```python
from build123d import *


with BuildPart() as f1:
    # F0 (on Front) → F1 (revolve)
    with BuildSketch(Plane.XZ):
        Polygon((0, 12.978721), (0, 0), (23.66708, 0), (23.66708, 56.037541), (65.809757, 64.282842), (65.809757, 75.581968), (50.235286, 75.581968), (-27.942425, 64.282842), (-27.942425, 56.037541), (0, 56.037541), (0, 47.486853), (-27.942425, 47.486853), (-27.942425, 39.546926), (0, 39.546926), (0, 30.080097), (-6.565706, 30.080097), (-6.565706, 21.224026), (-31.301621, 21.224026), (-31.301621, 12.978721), align=None)
    revolve(axis=Axis((11.83354, 0, 0), (-1, 0, 0)))


solid = f1.part
```
Read the model definition and answer for the solid it produces. Units are mm, in the model's axes. A direction names the side the tool comes from. Round coordinates to 2 decimals unless told otherwise and drop trailing zeros. Loops run counter-clockwise (first coordinate to the right, second up) from the corner with the lowest first, then second, coordinate; pieces in that order, holes last. Notation, with made-up numbers: (85.5, -37) -> (140.5, -37) arc R17 cw to (140.5, -29) -> close; hole circle Ø11 at (38.25, -28.5). An arc over 180 degrees is marked (long way). One line per item, written item: value.
1) Consider L1, parallel to Y at x = -11.75, z = 0; L2, parallel to Y at x = -7, z = -4.5; L3, parallel to Z at x = -26.5, y = 23. Determine where each line is inside the solid, lowest interval first. Write a range as [from, to].
Answer list:
L1: y = [-66.62, -56.04], [-47.49, -39.55], [-21.22, -12.98], [12.98, 21.22], [39.55, 47.49], [56.04, 66.62]
L2: y = [-67.16, -55.86], [-47.27, -39.29], [-20.74, -12.17], [12.17, 20.74], [39.29, 47.27], [55.86, 67.16]
L3: z = [-60.25, -51.1], [-41.55, -32.17], [32.17, 41.55], [51.1, 60.25]
2) The mould has two halves that part along Y. Classify faces 4 (the face through (-13.8, -38.6, -8.6)), 5 (the face through (-31.302, -9, -10)), 6 (the face through (57.914, -73.785, -16.385)): pulls with the +Y half, pulls with the -Y half, needs draft (parallel to the pull), parting line crosses it, or undercut.
Answer list:
face 4: undercut
face 5: needs draft
face 6: parting line crosses it
3) A cutting plane is placed at D-D (x = 14). Determine the outline of the cut face in (y, z), and give its area (3 significant figures).
Answer list:
outline: circle Ø140.69 at (0, 0)
area: 15,500 mm²
4) A cutting plane is placed at A-A (x = -12). Determine the outline of the cut face in (y, z), and give its area (3 significant figures).
Answer list:
outline: circle Ø133.17 at (0, 0); circle Ø94.97 at (0, 0); circle Ø42.45 at (0, 0); hole circle Ø112.08 at (0, 0); hole circle Ø79.09 at (0, 0); hole circle Ø25.96 at (0, 0)
area: 7,120 mm²
5) Flat-ended cylindrical pins translate along their axes: P1, Ø5, axis at x = 45.5, y = 17.5, coming from the -Z side; P2, Ø10, axis at x = -17.5, y = -25.5, coming from the +Z side; P3, Ø12, axis at y = -28, z = 30, coming from the -X side. Find the tip coordinate at first contact, or state that the pin passes through.
Answer list:
P1: stops at z = -73.5
P2: stops at z = 62.68
P3: stops at x = -27.94
6) For faces 1 (the face through (0, 13, -46)), 2 (the face through (65.81, 51, 40)), 3 (the face through (23.667, 1, 1)), determine the directions among +Z, -Z, +X, -X, +Y, -Y from which every point of the face is accessible in a straight line to the end or side of a thin tool.
Answer list:
face 1: -X
face 2: +Z, -Z, +X, +Y, -Y
face 3: +X
